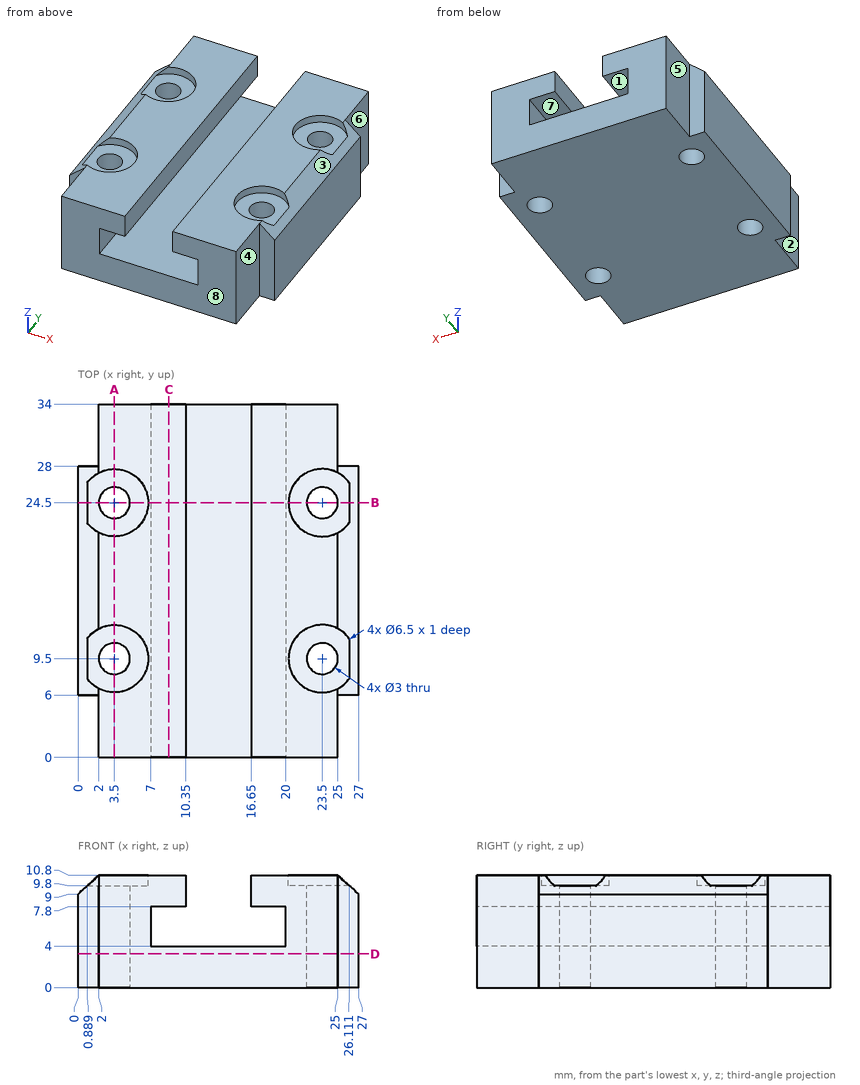
Job drawing, mm, ordinate dimensions from the low corner. One solid piece. A direction names the side the tool comes from. Give positions to 0.01 mm unless a question says otherwise; leave off trailing zeros. Loops run counter-clockwise (first coordinate to the right, second up) from the corner with the lowest first, then second, coordinate; pieces in that order, holes last. Notation, with made-up numbers: M 39.25,83.5 L 60.25,83.5 A14 cw 60.25,98.5 Z; hole C -23,-6 d6. An arc over 180 degrees is marked long. Put each result on its own line as item: value. Start each with the question number.
1) Saw through at B-B (y = 24.5). List the corners of the cut face in (x, z), then the cut area to 3 significant figures.
2) Pull direction X, two halves, no side cores. Call the marked faces 1, 2 and 3: +X half, -X half, draft (parallel to the pull), parting line (faces both ways), or undercut.
3) Flat gauge pins, fed straight in: pin 1 (3 mm diameter, centred on y = 10, z = 9, fed in from -X); pin 2 (1.5 mm diameter, centred on y = 25, z = 10, fed in from +X); pin 3 (1.6 mm diameter, centred on x = 26.5, z = 5.5, fed in from +Y); pin 4 (1.6 mm diameter, centred on x = 26.5, z = 7.5, fed in from -Y). Where does each tip first touch, or does it go through?
4) Saw through at D-D (z = 3.25). List the corners of the cut face in (x, y), then the cut area to 3 significant figures.
5) Probe probe 1 along Y at (x, z) = (23.5, 10.1); probe 2 along Y at (x, z) = (23.5, 3); probe 3 along Z at (x, y) = (9.75, 10). List the from-to ranges inside material, lowest first.
6) Saw through at C-C (x = 8.75). List the corners of the cut face in (y, z).
7) 3-axis set-ups, long thin cutter, end or side, ignore diameter. For the marked faces 4, 5, 6, 7 and 8: which of +Z, -Z, +X, -X, +Y, -Y reach the whole face in a straight line?
8) Saw through at A-A (x = 3.5). List the corners of the cut face in (y, z).
Numbers:
1. outline: M 0,0 L 2,0 L 2,9.8 L 0.89,9.8 L 0,9 Z; M 5,0 L 22,0 L 22,9.8 L 20.25,9.8 L 20.25,10.8 L 16.65,10.8 L 16.65,7.8 L 20,7.8 L 20,4 L 7,4 L 7,7.8 L 10.35,7.8 L 10.35,10.8 L 6.75,10.8 L 6.75,9.8 L 5,9.8 Z; M 25,0 L 27,0 L 27,9 L 26.11,9.8 L 25,9.8 Z
1. area: 150 mm^2
2. face 1: undercut
2. face 2: -X half
2. face 3: +X half
3. pin 1: x = 0
3. pin 2: x = 26.72
3. pin 3: y = 28
3. pin 4: y = 6
4. outline: M 0,6 L 2,6 L 2,0 L 25,0 L 25,6 L 27,6 L 27,28 L 25,28 L 25,34 L 2,34 L 2,28 L 0,28 Z; hole C 3.5,9.5 d3; hole C 3.5,24.5 d3; hole C 23.5,9.5 d3; hole C 23.5,24.5 d3
4. area: 842 mm^2
5. probe 1: 0 to 6.25, 12.75 to 21.25, 27.75 to 34
5. probe 2: 0 to 8, 11 to 23, 26 to 34
5. probe 3: 0 to 4, 7.8 to 10.8
6. outline: M 0,0 L 34,0 L 34,4 L 0,4 Z; M 0,7.8 L 34,7.8 L 34,10.8 L 0,10.8 Z
7. face 4: +Z, -Z, +X, -Y
7. face 5: +Z, -Z, -X, +Y
7. face 6: +Z, -Z, +X, +Y
7. face 7: +Y, -Y
7. face 8: +Z, -Z, +X, -X, -Y
8. outline: M 0,0 L 8,0 L 8,9.8 L 6.25,9.8 L 6.25,10.8 L 0,10.8 Z; M 11,0 L 23,0 L 23,9.8 L 21.25,9.8 L 21.25,10.8 L 12.75,10.8 L 12.75,9.8 L 11,9.8 Z; M 26,0 L 34,0 L 34,10.8 L 27.75,10.8 L 27.75,9.8 L 26,9.8 Z
